Input: dimensioned drawing with shaded views. Units: mm. Origin: part minimum x, y, z. A direction names the side the tool comes from. Round coordinates to 2 decimals unless told otherwise and drop trailing zeros. Order: outer loops, then holes, each group sorted by start corner. A loop starts at its lowest first (then second) coordinate and runs counter-clockwise, first axis right, second up.
Item 1: Line query: L1, parallel to Z at x = 33.5, y = 14.5; L2, parallel to X at y = 6.75, z = 23.75. Output: solid intervals per line, ascending.
Item 2: Cut plane A-A on x = 3.5. Output: boundary loops of the cut face in (y, z), then the cut area to 3 significant figures.
Item 3: First-contact query: pin 1 (10 mm diameter, centred on y = 3, z = 19, fed in from +X); pin 2 (10 mm diameter, centred on y = 5.5, z = 6.5, fed in from +X); pin 3 (4 mm diameter, centred on x = 22, z = 9, fed in from -Y). Flat tips, straight axial feed; report the tip coordinate or a pass-through.
Item 4: Cut plane D-D on x = 14. Output: boundary loops of the cut face in (y, z).
Item 5: Reachability of the marked faces 1, 2, 3, 4 and 5 from +Z, -Z, +X, -X, +Y, -Y: full face, straight path, thin tool, end or side. Return the list, or none.
Item 6: Cut plane C-C on z = 18.5. Output: boundary loops of the cut face in (x, y).
Item 7: Cut plane B-B on y = 9.5. Output: boundary loops of the cut face in (x, z), then the cut area to 3 significant figures.
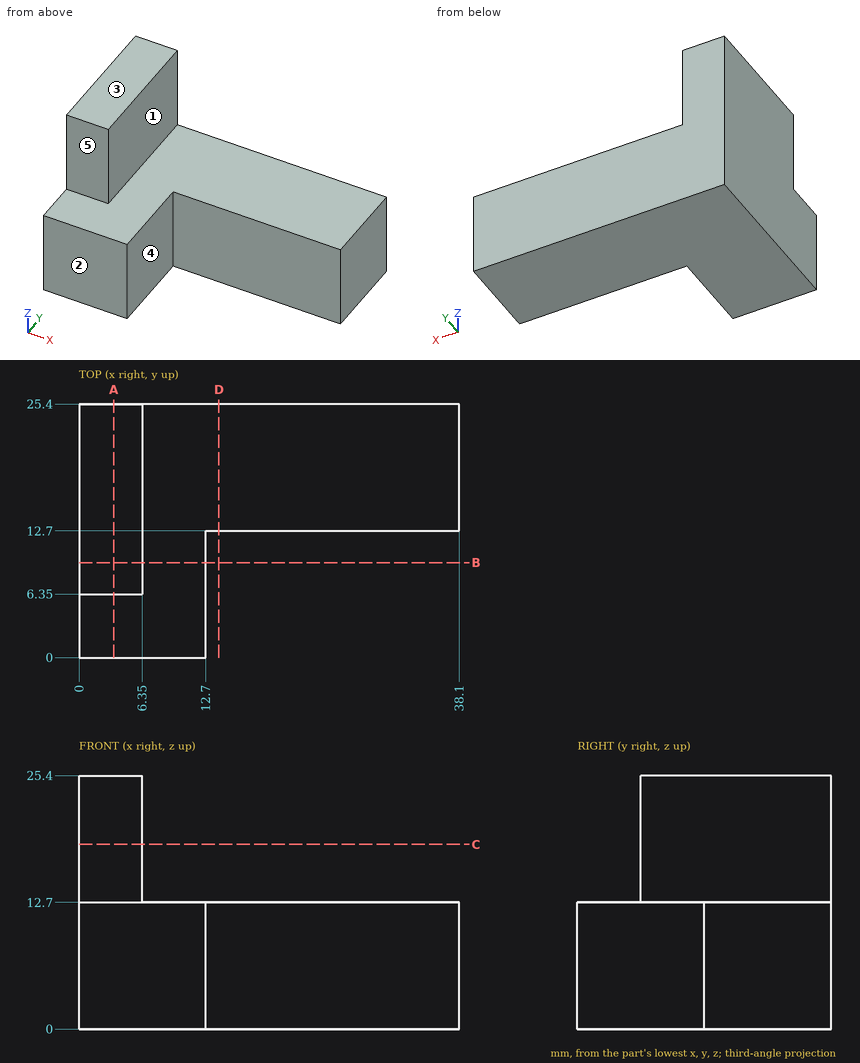
From the geometry:
1. L1: z = 0 to 12.7
1. L2: x = 0 to 6.35
2. outline: (0, 0) - (25.4, 0) - (25.4, 25.4) - (6.35, 25.4) - (6.35, 12.7) - (0, 12.7) - close
2. area: 565 mm2
3. pin 1: stops at x = 6.35
3. pin 2: stops at x = 12.7
3. pin 3: stops at y = 12.7
4. outline: (12.7, 0) - (25.4, 0) - (25.4, 12.7) - (12.7, 12.7) - close
5. face 1: +Z, +X, +Y, -Y
5. face 2: +Z, -Z, +X, -X, -Y
5. face 3: +Z, +X, -X, +Y, -Y
5. face 4: +Z, -Z, +X, -Y
5. face 5: +Z, +X, -X, -Y
6. outline: (0, 6.35) - (6.35, 6.35) - (6.35, 25.4) - (0, 25.4) - close
7. outline: (0, 0) - (12.7, 0) - (12.7, 12.7) - (6.35, 12.7) - (6.35, 25.4) - (0, 25.4) - close
7. area: 242 mm2
